Could you check a few things on this model? Use its own coordinates, in mm. A direction names the side the tool comes from. Coordinates: 2 decimals unless noted, no trailing zeros. Order: outer loops, then holes, each group sorted by start corner. A loop starts at its lowest first (then second) coordinate and runs counter-clockwise, first axis right, second up. Notation, with made-up numbers: (39, 38) - (66, 38) arc R24 cw to (66, 49) - close; hole circle Ø7 at (-8.75, 46.25). An arc over 180 degrees is marked (long way). Answer as a JSON object with one key per item and string values. Group by question number.
(1) Will these pins go through, and if not, where does the flat tip stop? P1, Ø8, axis at x = 11.5, y = 13.5, coming from the -Z side; P2, Ø1, axis at x = -11.5, z = -3.5, coming from the -Y side (3 decimals); P3, Ø1, axis at y = 14.5, z = 19.5, coming from the -X side.
(2) Imagine slicing it at A-A, the plane y = 0. Give the number of separate pieces and of enclosed holes in the cut face, and give its area (3 significant figures).
(3) Imagine slicing it at D-D, the plane y = 11.5. Write out the boundary of the cut face in (x, z) (3 decimals).
(4) Which directions (+Z, -Z, +X, -X, +Y, -Y) give clear straight access to the entire face, cutting with the end or side of a thin tool? Please do faces 1 (the cylindrical face through (-30.14, -0.62, 30.12)), 2 (the cylindrical face through (-13.858, -17.485, -10.626)), 3 (the cylindrical face through (-27.67, 14.92, 0.53)).
(5) We'd pull the mould along Y, two halves only. Please class faces 4 (the cylindrical face through (29.94, 17.14, 0.53)), 5 (the flat face through (0, -17, -38.1)), 6 (the cylindrical face through (30.18, -0.62, -20.68)), 7 (the flat face through (-6, -19.05, 17)): pulls with the +Y half, pulls with the -Y half, needs draft (parallel to the pull), parting line crosses it, or undercut.
(6) Imagine slicing it at C-C, the plane x = -20. Write out the boundary of the cut face in (y, z) (3 decimals), and give its area (3 significant figures).
(7) Please list where these lines run through material, in increasing order: probe 1 along Z at (x, y) = (-30.6, 0); probe 2 along Y at (x, z) = (13, -30.5) (3 decimals); probe 3 along X at (y, z) = (-10.5, 4) (3 decimals).
from build123d import *

# Parameters (mm, degrees)
F1_DEPTH = 38.1
F2_R     = 4.7625
F3_DEPTH = 63.501
F4_R     = 17.4625
F5_DEPTH = 3.175


with BuildPart() as f1:
    # F0 (on Top) → F1 (new body, symmetric)
    with BuildSketch(Plane.XY):
        with BuildLine():
            Line((-25.4, -19.05), (25.4, -19.05))
            ThreePointArc((25.4, -19.05), (29.890128, -17.190128), (31.75, -12.7))
            Line((31.75, -12.7), (31.75, 12.7))
            ThreePointArc((31.75, 12.7), (29.890128, 17.190128), (25.4, 19.05))
            Line((25.4, 19.05), (-25.4, 19.05))
            ThreePointArc((-25.4, 19.05), (-29.890128, 17.190128), (-31.75, 12.7))
            Line((-31.75, 12.7), (-31.75, -12.7))
            ThreePointArc((-31.75, -12.7), (-29.890128, -17.190128), (-25.4, -19.05))
        make_face()
        with BuildLine():
            Line((-25.4, 15.875), (25.4, 15.875))
            ThreePointArc((25.4, 15.875), (27.645064, 14.945064), (28.575, 12.7))
            Line((28.575, 12.7), (28.575, -12.7))
            ThreePointArc((28.575, -12.7), (27.645064, -14.945064), (25.4, -15.875))
            Line((25.4, -15.875), (-25.4, -15.875))
            ThreePointArc((-25.4, -15.875), (-27.645064, -14.945064), (-28.575, -12.7))
            Line((-28.575, -12.7), (-28.575, 12.7))
            ThreePointArc((-28.575, 12.7), (-27.645064, 14.945064), (-25.4, 15.875))
        make_face(mode=Mode.SUBTRACT)
    extrude(amount=F1_DEPTH, both=True)

    # F2 (on face) → F3 (cut, through all)
    with BuildSketch(Plane.YZ.offset(31.75)):
        with Locations((0, 25.4)):
            Circle(F2_R)
        with Locations((0, -25.4)):
            Circle(F2_R)
    extrude(amount=-F3_DEPTH, mode=Mode.SUBTRACT)

    # F4 (on face) → F5 (cut, through all)
    with BuildSketch(Plane.XZ.offset(19.05)):
        Circle(F4_R)
    extrude(amount=-F5_DEPTH, mode=Mode.SUBTRACT)


solid = f1.part
Result set:
{
 "1": {"P1": "stops at z = -38.1", "P2": "stops at y = 15.875", "P3": "stops at x = -31.62"},
 "2": {"separate pieces": "6", "enclosed holes": "0", "area": "363 mm^2"},
 "3": {"outline": "(-31.75, -38.1) - (-28.575, -38.1) - (-28.575, 38.1) - (-31.75, 38.1) - close; (28.575, -38.1) - (31.75, -38.1) - (31.75, 38.1) - (28.575, 38.1) - close"},
 "4": {"face 1": "+X, -X", "face 2": "-Y", "face 3": "+Z, -Z"},
 "5": {"face 4": "pulls with the +Y half", "face 5": "needs draft", "face 6": "undercut", "face 7": "pulls with the -Y half"},
 "6": {"outline": "(-19.05, -38.1) - (-15.875, -38.1) - (-15.875, 38.1) - (-19.05, 38.1) - close; (15.875, -38.1) - (19.05, -38.1) - (19.05, 38.1) - (15.875, 38.1) - close", "area": "484 mm^2"},
 "7": {"probe 1": "z = -38.1 to -30.16, -20.64 to 20.64, 30.16 to 38.1", "probe 2": "y = -19.05 to -15.875, 15.875 to 19.05", "probe 3": "x = -31.75 to -28.575, 28.575 to 31.75"}
}
